Design review of the part shown in the three views and the two pictorial views. Dimensions are in mm from the part's minimum x, y and z. Coordinates: 2 decimals unless noted, no trailing zeros. Write each loop counter-clockwise with the first axis right and the second up, starting at its lowest first coordinate (ties: lowest second). Pieces come first, ordered by that corner, then holes. Notation, with made-up numbers: (51.25, 17.5) -> (91.25, 17.5) arc R34 ccw to (91.25, 50.5) -> close; hole circle Ø8 at (31.5, 37.5). An arc over 180 degrees is marked (long way). Answer in a Markdown table with one row per item. Add a question column.
Item 1: Take a section at B-B, the plane y = 68. Write out the cut boundary in (x, z), and give its area (3 significant figures).
Item 2: Take a section at A-A, the plane x = 91.5. Write out the cut boundary in (y, z) (1 decimal), and give its area (3 significant figures).
Item 3: Clearance check with a flat-ended pin moving along its axis: P1, Ø3, axis at x = 220, y = 61, coming from the +Z side. State where the tip first meets the part, or that it passes through.
Item 4: To check wall thickness, follow line 1 (X direction, y = 313.5, z = 5.25); line 2 (Y direction, x = 357.5, z = 4.75) (1 decimal). State the ranges of each line that lie inside material, in increasing order.
Item 5: Take a section at C-C, the plane z = 7.75. Write out the cut boundary in (x, y) (1 decimal), and give its area (3 significant figures).
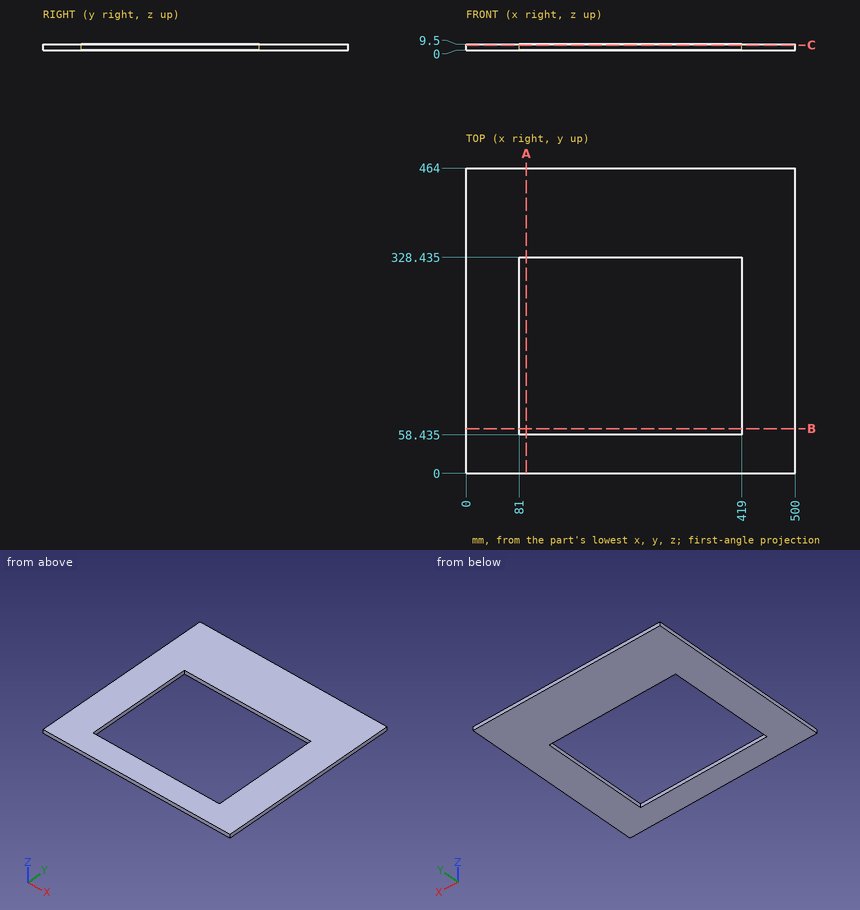
Answers:
| question | item | result |
|---|---|---|
| 1 | outline | (0, 0) -> (81, 0) -> (81, 9.5) -> (0, 9.5) -> close; (419, 0) -> (500, 0) -> (500, 9.5) -> (419, 9.5) -> close |
| 1 | area | 1,540 mm^2 |
| 2 | outline | (0, 0) -> (58.4, 0) -> (58.4, 9.5) -> (0, 9.5) -> close; (328.4, 0) -> (464, 0) -> (464, 9.5) -> (328.4, 9.5) -> close |
| 2 | area | 1,840 mm^2 |
| 3 | P1 | passes through |
| 4 | line 1 | x = 0 to 81, 419 to 500 |
| 4 | line 2 | y = 0 to 58.4, 328.4 to 464 |
| 5 | outline | (0, 0) -> (500, 0) -> (500, 464) -> (0, 464) -> close; hole (81, 58.4) -> (419, 58.4) -> (419, 328.4) -> (81, 328.4) -> close |
| 5 | area | 141,000 mm^2 |
